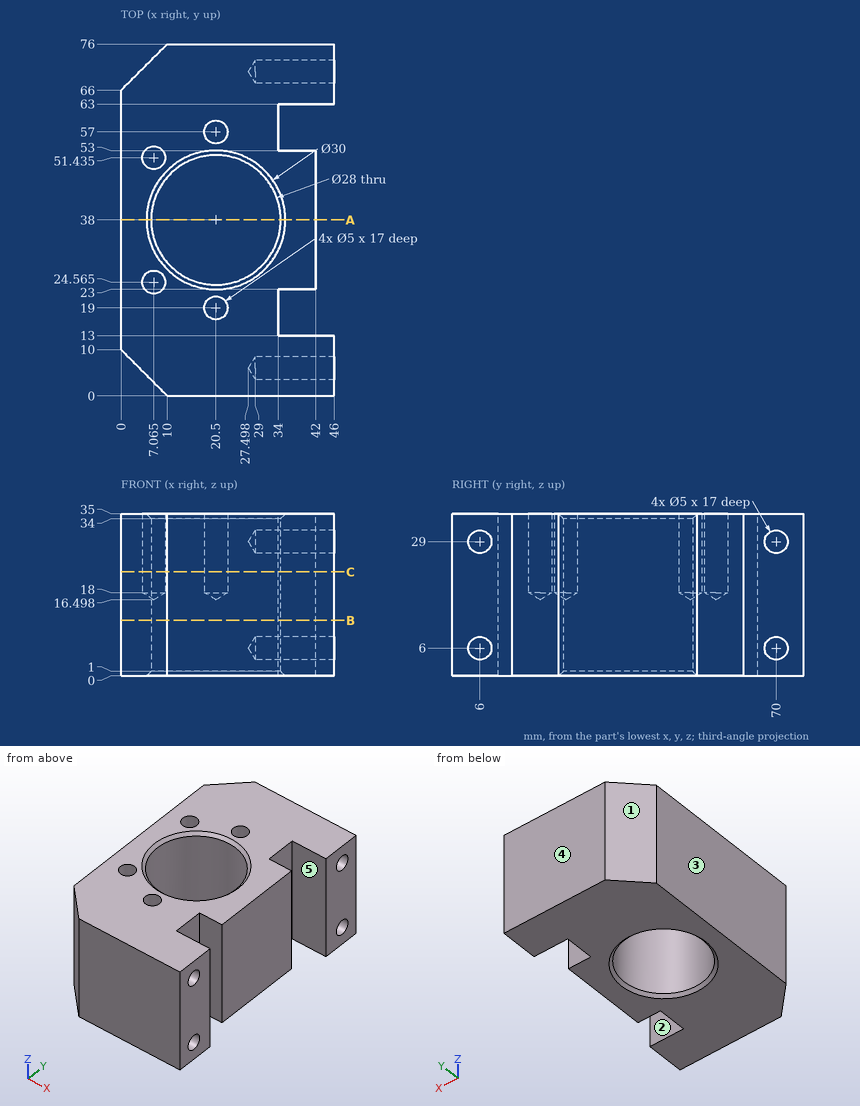
The drawing under review shows one solid part. Ordinate dimensions are in mm from its lowest x, y, z. A direction names the side the tool comes from. Round coordinates to 2 decimals unless told otherwise and drop trailing zeros. Loops run counter-clockwise (first coordinate to the right, second up) from the corner with the lowest first, then second, coordinate; pieces in that order, holes last. Notation, with made-up numbers: (-37, 82) - (1, 82) arc R16 ccw to (1, 92) - close; hole circle Ø4 at (68.25, 62). An arc over 180 degrees is marked (long way). Use one line per item in the form item = value.
Item 1: Clearance check with flat-ended pins moving along their axes: P1, Ø4, axis at y = 6, z = 29, coming from the +X side; P2, Ø12, axis at y = 28, z = 15.5, coming from the +X side; P3, Ø4.5, axis at x = 7.06, y = 51.44, coming from the +Z side. State where each tip first meets the part, or that it passes through.
Answers:
P1 = 28.7
P2 = 42
P3 = 17.85
Item 2: Consider section A-A on y = 38. Write out the cut boundary in (x, z), then the cut area to 3 significant figures.
Answers:
outline = (0, 0) - (5.5, 0) - (6.5, 1) - (6.5, 34) - (5.5, 35) - (0, 35) - close; (34.5, 1) - (35.5, 0) - (42, 0) - (42, 35) - (35.5, 35) - (34.5, 34) - close
area = 488 mm^2
Item 3: Tool access review of the marked faces 1 and 2: name each direction out of +Z, -Z, +X, -X, +Y, -Y from which nothing blocks a thin tool from reaching the whole face with its end or side.
Answers:
face_1 = +Z, -Z, -X, +Y
face_2 = +Z, -Z, +X
Item 4: Consider section C-C on z = 22.5. Write out the cut boundary in (x, y) (3 decimals).
Answers:
outline = (0, 10) - (10, 0) - (46, 0) - (46, 13) - (34, 13) - (34, 23) - (42, 23) - (42, 53) - (34, 53) - (34, 63) - (46, 63) - (46, 76) - (10, 76) - (0, 66) - close; hole circle Ø5 at (7.065, 24.565); hole circle Ø5 at (7.065, 51.435); hole circle Ø28 at (20.5, 38); hole circle Ø5 at (20.5, 19); hole circle Ø5 at (20.5, 57)
Item 5: Mouldability with a two-part tool opening along Y and no side actions: class the marked faces 3, 4 and 5 as +Y half, -Y half, draft (parallel to the pull), parting line (faces both ways), or undercut.
Answers:
face_3 = draft
face_4 = +Y half
face_5 = undercut
Item 6: For line 1 (Y direction, x = 40.5, z = 6); line 2 (Z direction, x = 42.5, y = 6); line 3 (Y direction, x = 19, z = 25.5), list the stretches that pass through material, from the lowest coordinate up.
Answers:
line_1 = 0 to 3.5, 8.5 to 13, 23 to 53, 63 to 67.5, 72.5 to 76
line_2 = 0 to 3.5, 8.5 to 26.5, 31.5 to 35
line_3 = 0 to 17, 21 to 24.08, 51.92 to 55, 59 to 76
Item 7: Consider section B-B on z = 12. Write out the cut boundary in (x, y), then the cut area to 3 significant figures.
Answers:
outline = (0, 10) - (10, 0) - (46, 0) - (46, 13) - (34, 13) - (34, 23) - (42, 23) - (42, 53) - (34, 53) - (34, 63) - (46, 63) - (46, 76) - (10, 76) - (0, 66) - close; hole circle Ø28 at (20.5, 38)
area = 2,420 mm^2
